```python
from build123d import *

# Parameters (mm, degrees)
BOSS_EXTRUDE2_DEPTH = 30
BOSS_EXTRUDE3_DEPTH = 5
BOSS_EXTRUDE4_DEPTH = 5
SKETCH4_R           = 1.5
CUT_EXTRUDE1_DEPTH  = 46
SKETCH5_R           = 1.5
CUT_EXTRUDE2_DEPTH  = 6
FILLET1_R           = 2
FILLET2_R           = 5


with BuildPart() as part:
    # Sketch1 → Boss-Extrude2 (new body)
    with BuildSketch(Plane.XY):
        Polygon((0, 0), (0, 45), (5, 45), (5, 5), (45, 5), (45, 0), align=None)
    extrude(amount=BOSS_EXTRUDE2_DEPTH)

    # Sketch2 → Boss-Extrude3 (add)
    with BuildSketch(Plane.XY.offset(30)):
        Polygon((5, 45), (45, 5), (5, 5), align=None)
    extrude(amount=-BOSS_EXTRUDE3_DEPTH)

    # Sketch3 → Boss-Extrude4 (add)
    with BuildSketch(Plane(origin=(0, 0, 0), x_dir=(-1, 0, 0), z_dir=(0, 0, -1))):
        Polygon((-5, 45), (-5, 5), (-45, 5), align=None)
    extrude(amount=-BOSS_EXTRUDE4_DEPTH)

    # Sketch4 → Cut-Extrude1 (cut, through all)
    with BuildSketch(Plane.XZ):
        with Locations((15, 15)):
            Circle(SKETCH4_R)
    extrude(amount=-CUT_EXTRUDE1_DEPTH, mode=Mode.SUBTRACT)

    # Sketch5 → Cut-Extrude2 (cut, through all)
    with BuildSketch(Plane.XY.offset(5)):
        with Locations((15, 15)):
            Circle(SKETCH5_R)
    extrude(amount=-CUT_EXTRUDE2_DEPTH, mode=Mode.SUBTRACT)

    # Fillet1
    fillet1_edges = [part.edges().sort_by_distance(p)[0] for p in [
        (0, 45, 15),
        (45, 0, 15),
        (25, 25, 30),
        (25, 25, 0),
    ]]
    fillet(fillet1_edges, radius=FILLET1_R)

    # Fillet2
    fillet2_edges = [part.edges().sort_by_distance(p)[0] for p in [
        (0, 0, 15),
    ]]
    fillet(fillet2_edges, radius=FILLET2_R)


solid = part.part
```
Input: part model. Units: mm. Frame: model coordinates. A direction names the side the tool comes from. Coordinates: 2 decimals unless noted, no trailing zeros. Write each loop counter-clockwise with the first axis right and the second up, starting at its lowest first coordinate (ties: lowest second). Pieces come first, ordered by that corner, then holes. Notation, with made-up numbers: (5, 42.5) - (57, 42.5) arc R18 ccw to (57, 49.5) - close; hole circle Ø5 at (81, 77.5). An arc over 180 degrees is marked (long way). Put each result on its own line as item: value. Start each with the question number.
1) Cut plane A-A (z = 15). Return the cut outline in (x, y).
2) Cut plane C-C (z = 11.75). Return the cut outline in (x, y), plus the area to 3 significant figures.
3) Mould query, pull axis Z, two halves, no side actions, for faces 4 (the face through (5, 25, 15)), 5 (the face through (24.297, 24.897, 0.601)), 6 (the face through (0, 24, 15)). Classes: pulls with the +Z half, pulls with the -Z half, needs draft (parallel to the pull), parting line crosses it, or undercut.
4) Reachability of faces 1 (the face through (20, 16, 5)), 2 (the face through (2, 1, 15)), 3 (the face through (13.5, 15.07, 2.54)) from +Z, -Z, +X, -X, +Y, -Y: full face, straight path, thin tool, end or side. Return the list, or none.
5) Ray query, L1, parallel to Z at x = 20, y = 17.5; L2, parallel to Z at x = 15, y = 2.7; L3, parallel to Y at x = 15, z = 1.3. Return the intervals inside material, ascending.
6) Cut plane D-D (x = 15). State how many separate pieces and enclosed holes the cut face has, plus the area to 3 significant figures.
7) Contact query for flat-ended pins moving along their axis: pin 1 (20 mm diameter, centred on x = 29.5, y = 31, fed in from +Z); pin 2 (4 mm diameter, centred on x = 10, z = 23.5, fed in from +Y); pin 3 (6 mm diameter, centred on x = 32, z = 9, fed in from +Y); pin 4 (12 mm diameter, centred on x = 33, y = 27, fed in from +Z). Output: stop coordinate, or through.
8) Cut plane B-B (z = 3). Return the cut outline in (x, y), plus the area to 3 significant figures.
Resolved:
1. outline: (0, 5) arc R5 ccw to (5, 0) - (13.5, 0) - (13.5, 5) - (5, 5) - (5, 45) - (2, 45) arc R2 ccw to (0, 43) - close; (16.5, 0) - (43, 0) arc R2 ccw to (45, 2) - (45, 5) - (16.5, 5) - close
2. outline: (0, 5) arc R5 ccw to (5, 0) - (43, 0) arc R2 ccw to (45, 2) - (45, 5) - (5, 5) - (5, 45) - (2, 45) arc R2 ccw to (0, 43) - close
2. area: 418 mm2
3. face 4: undercut
3. face 5: pulls with the -Z half
3. face 6: needs draft
4. face 1: +X, +Y
4. face 2: +Z, -Z, -X, -Y
4. face 3: -Z
5. L1: z = 0 to 5, 25 to 30
5. L2: z = 0 to 13.5, 16.5 to 30
5. L3: y = 0 to 13.5, 16.5 to 34.82
6. separate pieces: 3
6. enclosed holes: 0
6. area: 418 mm2
7. pin 1: stops at z = 30
7. pin 2: stops at y = 41.32
7. pin 3: stops at y = 5
7. pin 4: passes through
8. outline: (0, 5) arc R5 ccw to (5, 0) - (43, 0) arc R2 ccw to (45, 2) - (45, 5) - (5, 45) - (2, 45) arc R2 ccw to (0, 43) - close; hole circle Ø3 at (15, 15)
8. area: 1,210 mm2
